Read the model definition and answer for the solid it produces. Units are mm, in the model's axes. Face numbers are marked on the shaded views. A direction names the side the tool comes from. Give positions to 0.01 mm unless a question says otherwise; leave off trailing zeros. Loops run counter-clockwise (first coordinate to the right, second up) from the corner with the lowest first, then second, coordinate; pieces in that order, holes last. Notation, with made-up numbers: (19.25, -38.75) - (54.25, -38.75) arc R18 ccw to (54.25, -19.75) - close; hole circle Ø8 at (-34.5, -4). An arc over 180 degrees is marked (long way). Write each question's results on one line, items separated by ' | '. Start each with the question number.
Q1. The part is cut by section A-A, the plane z = 41. Write down the section's boundary in (x, y).
Q2. Given pin 1 (10 mm diameter, centred on x = 42, z = 27, fed in from -Y); pin 2 (6 mm diameter, centred on x = 62, z = 29.5, fed in from +Y); pin 3 (1.5 mm diameter, centred on x = 53.5, z = 32, fed in from +Y), each flat-ended and moving along its own axis, determine where each tip first touches the part or whether it passes through.
Q3. The part is cut by section B-B, the plane y = -8. Write down the section's boundary in (x, z).
Q4. Determine the mould class of the marked faces 1, 2 and 3 for opening direction X: +X half, -X half, draft (parallel to the pull), parting line (faces both ways), or undercut.
Q5. The part is cut by section D-D, the plane z = 34. Write down the section's boundary in (x, y).
Q6. Find the intervals of material crossed by line 1 (X direction, y = -45, z = 6); line 2 (Y direction, x = 7, z = 26); line 3 (Z direction, x = -3.5, y = -6.5), in increasing order. Write a range as from..to.
Q7. The part is cut by section C-C, the plane x = -3. Write down the section's boundary in (y, z).
Q8. For the marked faces 4, 5 and 6, determine the directions among +Z, -Z, +X, -X, +Y, -Y from which every point of the face is accessible in a straight line to the end or side of a thin tool.
```python
from build123d import *

# Parameters (mm, degrees)
EXTRUDE_1_DEPTH = 1
DRAFT_5_ANGLE   = 43


with BuildPart() as part:
    # 草图1 → 凸台-拉伸1 (new body)
    with BuildSketch(Plane.XY):
        Polygon((-9.644281244, 0), (30.355718756, 0), (30.355718756, -10), (50.355718756, -10), (50.355718756, 0), (70.355718756, 0), (70.355718756, -50), (50.355718756, -50), (50.355718756, -40), (30.355718756, -40), (30.355718756, -50), (-9.644281244, -50), align=None)
    extrude(amount=EXTRUDE_1_DEPTH)

    # 拔模5
    draft_5_faces = [part.faces().sort_by_distance(p)[0] for p in [
        (29.244607645, -25, 1),
    ]]
    draft(draft_5_faces, Plane(origin=(-9.644281244, 0, 1), x_dir=(1, 0, 0), z_dir=(0, 1, 0)), DRAFT_5_ANGLE)


solid = part.part
```
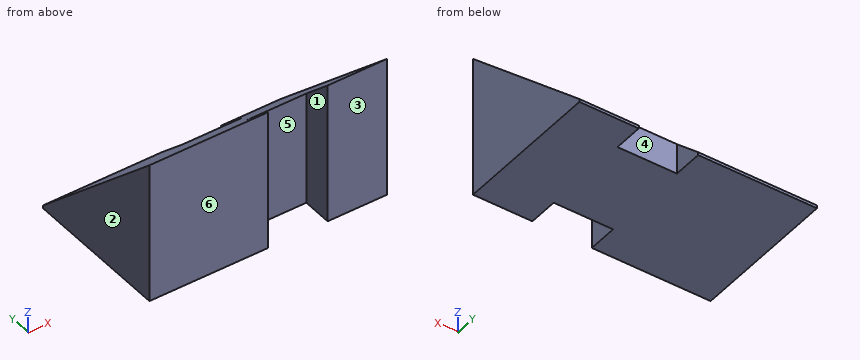
Check sheet entries:
1) outline: (-9.64, -50) - (30.36, -50) - (30.36, -42.89) - (-9.64, -42.89) - close; (50.36, -50) - (70.36, -50) - (70.36, -42.89) - (50.36, -42.89) - close
2) pin 1: stops at y = -40 | pin 2: stops at y = -27.35 | pin 3: stops at y = -32.44
3) outline: (-9.64, 0) - (30.36, 0) - (30.36, 8.46) - (-9.64, 8.46) - close; (50.36, 0) - (70.36, 0) - (70.36, 8.46) - (50.36, 8.46) - close
4) face 1: undercut | face 2: -X half | face 3: draft
5) outline: (-9.64, -50) - (30.36, -50) - (30.36, -40) - (50.36, -40) - (50.36, -50) - (70.36, -50) - (70.36, -35.39) - (-9.64, -35.39) - close
6) line 1: x = -9.64..30.36, 50.36..70.36 | line 2: y = -50..-26.81 | line 3: z = 0..7.06
7) outline: (-50, 0) - (0, 0) - (0, 1) - (-50, 47.63) - close
8) face 4: +Z, -Z, +Y | face 5: +Z, -Z, -Y | face 6: +Z, -Z, +X, -X, -Y
